The figure shows three views and two pictorial views of one solid part (mm, origin at its lowest corner). Answer the questions. A direction names the side the tool comes from. Round coordinates to 2 decimals unless told otherwise and drop trailing zeros. Order: outer loops, then holes, each group sorted by start corner. A loop starts at its lowest first (then second) coordinate and runs counter-clockwise, first axis right, second up. Notation, with made-up numbers: (32.25, 0.5) - (38.25, 0.5) arc R24 ccw to (38.25, 31.5) - close; hole circle Ø1 at (48, 34). An arc over 180 degrees is marked (long way). Use CSV: the item, a comma, the result in double quotes.
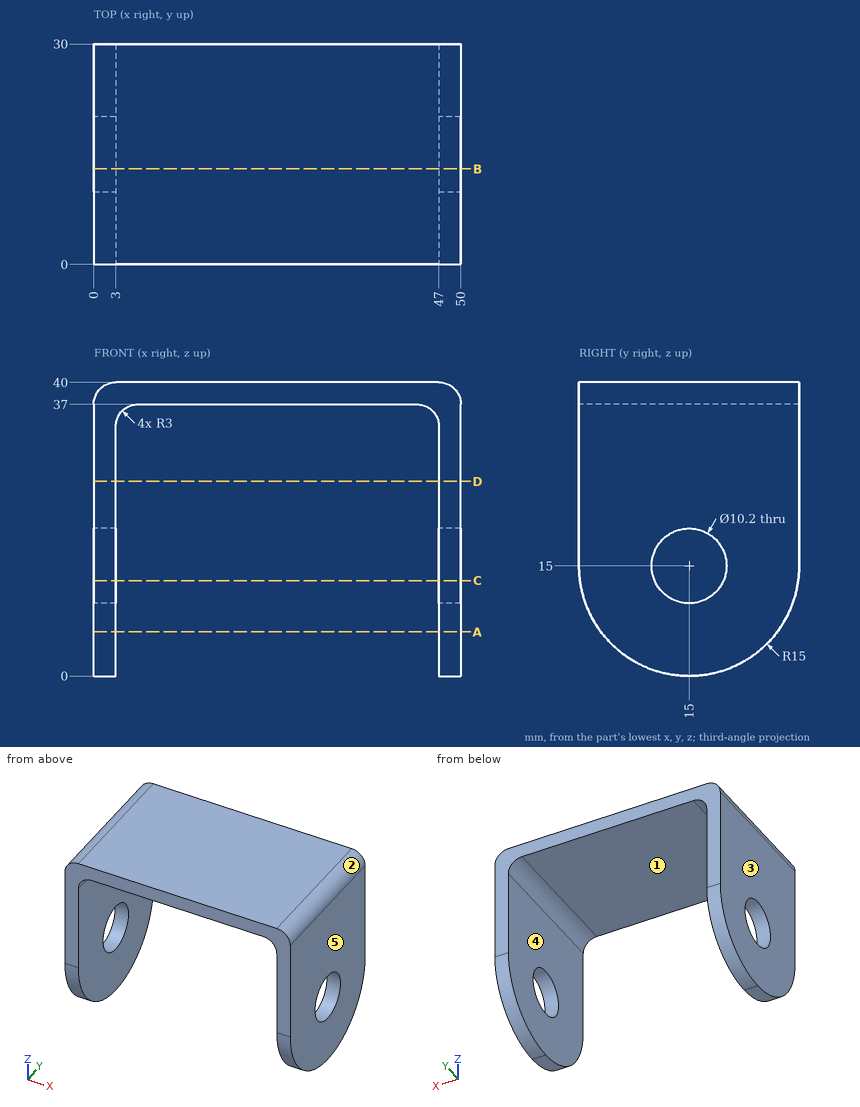
(1) Find section A-A (z = 6). Determine the outline of the cut face in (x, y).
Findings below:
outline,"(0, 3) - (3, 3) - (3, 27) - (0, 27) - close; (47, 3) - (50, 3) - (50, 27) - (47, 27) - close"
(2) Find section B-B (y = 13). Determine the outline of the cut face in (x, z), and give its area (3 significant figures).
Findings below:
outline,"(0, 0.13) - (3, 0.13) - (3, 10.31) - (0, 10.31) - close; (0, 19.69) - (3, 19.69) - (3, 34) arc R3 cw to (6, 37) - (44, 37) arc R3 cw to (47, 34) - (47, 19.69) - (50, 19.69) - (50, 37) arc R3 ccw to (47, 40) - (3, 40) arc R3 ccw to (0, 37) - close; (47, 0.13) - (50, 0.13) - (50, 10.31) - (47, 10.31) - close"
area,"315 mm²"
(3) Find section C-C (z = 13). Determine the outline of the cut face in (x, y), and give its area (3 significant figures).
Findings below:
outline,"(0, 0.13) - (3, 0.13) - (3, 10.31) - (0, 10.31) - close; (0, 19.69) - (3, 19.69) - (3, 29.87) - (0, 29.87) - close; (47, 0.13) - (50, 0.13) - (50, 10.31) - (47, 10.31) - close; (47, 19.69) - (50, 19.69) - (50, 29.87) - (47, 29.87) - close"
area,"122 mm²"
(4) The mould has two halves that part along X. Classify the marked faces 1, 2 and 3: released by +X, released by -X, zero draft, split by the parting line, or undercut.
Findings below:
face 1,"undercut"
face 2,"released by +X"
face 3,"released by -X"
(5) This flat-tipped pin is pushed along its axis until it touches: pin 1 (10 mm diameter, centred on x = 28, y = 21, fed in from -Z). Where does it stop, or does it pass through?
Findings below:
pin 1,"stops at z = 37"
(6) For the marked faces 4 and 5, determine the directions among +Z, -Z, +X, -X, +Y, -Y from which every point of the face is accessible in a straight line to the end or side of a thin tool.
Findings below:
face 4,"-Z, +Y, -Y"
face 5,"+Z, -Z, +X, +Y, -Y"
(7) Find the intervals of material crossed by L1, parallel to X at y = 10.5, z = 27; L2, parallel to X at y = 23, z = 36.5; L3, parallel to Z at x = 49.45, y = 15, in increasing order. Write a range as from..to.
Findings below:
L1,"x = 0..3, 47..50"
L2,"x = 0..4.34, 45.66..50"
L3,"z = 0..9.9, 20.1..38.73"
(8) Find section D-D (z = 26.5). Determine the outline of the cut face in (x, y).
Findings below:
outline,"(0, 0) - (3, 0) - (3, 30) - (0, 30) - close; (47, 0) - (50, 0) - (50, 30) - (47, 30) - close"
